from build123d import *

# Parameters (mm, degrees)
F1_DEPTH  = 3.175
F3_DEPTH  = 10.16
F5_DEPTH  = 21.4507239097
F6_COUNT  = 3
F8_DEPTH  = 9.5
F10_DEPTH = 9.5


with BuildPart() as f1:
    # F0 (on Front) → F1 (new body, symmetric)
    with BuildSketch(Plane.XZ):
        Polygon((0, -5.485), (0, -6.985), (2.625, -6.985), (2.625, -14.985), (26.9478585707, -14.985), (46.8930374778, -1.2901832047), (41.1420940815, 7.0855107996), (33.7226801014, 1.9911711769), (22.8343583448, -5.485), align=None)
    extrude(amount=F1_DEPTH, both=True)

    # F2 (on face) → F3 (join, through all)
    with BuildSketch(Plane(origin=(9.8755636575, 0, -14.3828053272), x_dir=(0.8243793311, 0, 0.5660377358), z_dir=(-0.5660377358, 0, 0.8243793311))):
        with BuildLine():
            Line((30.23841274, 3.175), (36.6163042411, 3.175))
            ThreePointArc((36.6163042411, 3.175), (33.4273584906, 4.5), (30.23841274, 3.175))
        make_face()
        with BuildLine():
            ThreePointArc((30.23841274, -3.175), (33.4273584906, -4.5), (36.6163042411, -3.175))
            Line((36.6163042411, -3.175), (30.23841274, -3.175))
        make_face()
        with BuildLine():
            ThreePointArc((36.6163042411, -3.175), (37.5867007389, -1.7175191589), (37.9273584906, 0))
            ThreePointArc((37.9273584906, 0), (37.5867007389, 1.7175191589), (36.6163042411, 3.175))
            Line((36.6163042411, 3.175), (30.23841274, 3.175))
            ThreePointArc((30.23841274, 3.175), (28.9273584906, 0), (30.23841274, -3.175))
            Line((30.23841274, -3.175), (36.6163042411, -3.175))
        make_face()
    extrude(amount=-F3_DEPTH)

    # F4 (on face) → F5 (cut, through all)
    with BuildSketch(Plane(origin=(9.8755636575, 0, -14.3828053272), x_dir=(0.8243793311, 0, 0.5660377358), z_dir=(-0.5660377358, 0, 0.8243793311))):
        with BuildLine():
            Line((36.6163042411, -3.175), (37.9273584906, -3.175))
            Line((37.9273584906, -3.175), (37.9273584906, 0))
            ThreePointArc((37.9273584905, 0), (37.5867007389, -1.7175191589), (36.6163042411, -3.175))
        make_face()
        with BuildLine():
            ThreePointArc((36.6163042411, 3.175), (37.5867007389, 1.7175191589), (37.9273584905, 0))
            Line((37.9273584906, 0), (37.9273584906, 3.175))
            Line((37.9273584906, 3.175), (36.6163042411, 3.175))
        make_face()
    extrude(amount=-F5_DEPTH, mode=Mode.SUBTRACT)

    # F6: F1 ×3 about axis
    f6_axis = Axis((0, 0, -2.7425), (0, 0, -1))


with BuildPart() as f1_1:
    add(f1.part)
    for i in range(1, F6_COUNT):
        add(f1.part.rotate(f6_axis, i * 360 / F6_COUNT))

    # F7 (on face) → F8 (join, through all)
    with BuildSketch(Plane(origin=(0, 0, -14.985), x_dir=(1, 0, 0), z_dir=(0, 0, -1))):
        with BuildLine():
            ThreePointArc((-1.3124999835, 2.2733166945), (1.3125000082, 2.2733166802), (2.625, 0))
            Line((2.625, 0), (2.625, 3.175))
            Line((2.625, 3.175), (3.965573729, 3.175))
            ThreePointArc((3.965573729, 3.175), (2.54, 4.3994090512), (0.7668437925, 5.0217875899))
            Line((0.7668437925, 5.0217875899), (1.437130657, 3.8608166849))
            Line((1.437130657, 3.8608166849), (-1.3124999835, 2.2733166945))
        make_face()
        with BuildLine():
            Line((2.625, -3.175), (2.625, 0))
            ThreePointArc((2.625, 0), (-1.3125000082, -2.2733166802), (-1.3124999835, 2.2733166945))
            Line((-1.3124999835, 2.2733166945), (-4.062130657, 0.6858166849))
            Line((-4.062130657, 0.6858166849), (-4.7324175215, 1.8467875899))
            ThreePointArc((-4.7324175215, 1.8467875899), (-2.54, -4.3994090512), (3.965573729, -3.175))
            Line((3.965573729, -3.175), (2.625, -3.175))
        make_face()
    extrude(amount=-F8_DEPTH)

    # F9 (on face) → F10 (join, through all)
    with BuildSketch(Plane(origin=(0, 0, -14.985), x_dir=(1, 0, 0), z_dir=(0, 0, -1))):
        with BuildLine():
            ThreePointArc((2.25, -1.3520817283), (2.5295132931, -0.70156076), (2.625, 0))
            ThreePointArc((2.625, 0), (2.5295132931, 0.70156076), (2.25, 1.3520817283))
            Line((2.25, 1.3520817283), (2.25, -1.3520817283))
        make_face()
    extrude(amount=-F10_DEPTH)


solid = f1_1.part
Check sheet for the modelled part. Datum: model origin and axes. Units: mm. A direction names the side the tool comes from. Give positions to 0.01 mm unless a question says otherwise; leave off trailing zeros. Loops run counter-clockwise (first coordinate to the right, second up) from the corner with the lowest first, then second, coordinate; pieces in that order, holes last. Notation, with made-up numbers: M 13,46 L 26,46 A24 cw 26,74 Z; hole C -6.75,-5.75 d9. An arc over 180 degrees is marked long. Return JSON: item names as keys, results as strings. Group by question number.
1. Go/stop test with flat-tipped pins: pin 1 (6 mm diameter, centred on y = -30.5, z = 0.5, fed in from -X); pin 2 (4 mm diameter, centred on x = 0, y = 0, fed in from +Z) (3 decimals); pin 3 (12 mm diameter, centred on y = -29.5, z = -5, fed in from -X). Record where each tip stops, or that it passes through.
2. Cross-section at B-B on x = 14. Record the boundary of the cut face in (y, z) (3 decimals).
3. Cross-section at A-A on z = 0.5. State how many separate pieces and enclosed holes the cut face has, plus the area to 3 significant figures.
4. Tool access check on faces 1 (the cylindrical face through (-5.08, -0.03, -10.3)), 2 (the flat face through (2.25, 0, -11)). Record the directions out of +Z, -Z, +X, -X, +Y, -Y that give a thin tool (end or side, any length) a straight path to the whole face; none if there is none.
5. Thickness scan on L1, parallel to Y at x = 0, z = -10.5 (3 decimals); L2, parallel to Z at x = 15, y = 0 (3 decimals); L3, parallel to Y at x = 11, z = -11.5 (3 decimals). Record the ranges inside material, lowest first.
6. Mould release check, pull along Y, two halves, no side actions. Record for faces 3 (the flat face through (-3, 0, -14.985)), 4 (the cylindrical face through (2.56, -4.39, -10.3)), 5 (the flat face through (-13.752, 17.468, -7.971)): released by +Y, released by -Y, zero draft, split by the parting line, or undercut.
7. Cross-section at C-C on y = -9. Record the boundary of the cut face in (x, z) (3 decimals), plus the area to 3 significant figures.
Return value:
{
 "1": {"pin 1": "x = -24.47", "pin 2": "z = -5.485", "pin 3": "x = -25.6"},
 "2": {"outline": "M -3.175,-14.985 L 3.175,-14.985 L 3.175,-5.485 L -3.175,-5.485 Z"},
 "3": {"separate pieces": "3", "enclosed holes": "0", "area": "302 mm^2"},
 "4": {"face 1": "+Z, -Z, -X", "face 2": "-Z"},
 "5": {"L1": "-6.35 to -2.625, 2.625 to 6.35", "L2": "-14.985 to -5.485", "L3": "-3.175 to 3.175"},
 "6": {"face 3": "zero draft", "face 4": "released by -Y", "face 5": "undercut"},
 "7": {"outline": "M -8.862,-14.985 L -1.53,-14.985 L -1.53,-5.485 L -8.862,-5.485 Z", "area": "69.7 mm^2"}
}
